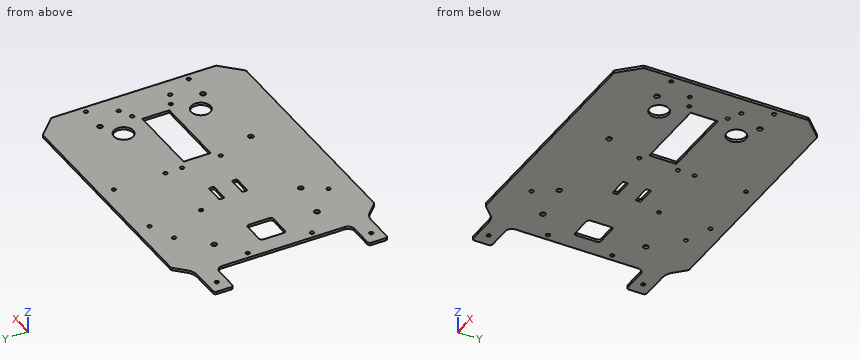
Autodesk Inventor part; units mm, degrees
ref_plane "РабПлоскость1" through (24.5, 0, 0) normal (0, 1, 0) x (1, 0, 0)
ref_plane "YZ Plane" through (0, 0, 0) normal (1, 0, 0) x (0, 1, 0)
ref_plane "XZ Plane" through (0, 0, 0) normal (0, 1, 0) x (-1, 0, 0)
sketch "Эскиз1" plane through (0, 0, 0) normal (0, 0, 1) x (1, 0, 0)
  line L0 (105, -79) -> (-105, -79)
  line L1 (-105, -79) -> (-105, 79)
  line L2 (-105, 79) -> (105, 79)
  line L3 (105, 79) -> (105, -79)
  line L4 (105, -79) -> (-105, 79) construction
  line L5 (-105, -79) -> (105, 79) construction
  point P0 (0, 0)
  dimension "d0" = 210
  dimension "d1" = 158
extrude "Выдавливание1" add sketch "Эскиз1" along normal blind 2
chamfer "Фаска1" distance 15 angle 45 4 edges at (105, -79, 1) (-105, -79, 1) (-105, 79, 1) (105, 79, 1)
fillet "Сопряжение1" radius 2 8 edges at (90, 79, 1) (105, 64, 1) (105, -64, 1) (90, -79, 1) (-90, -79, 1) (-105, -64, 1) (-90, 79, 1) (-105, 64, 1)
sketch "Эскиз2" plane through (0, 0, 2) normal (0, 0, 1) x (1, 0, 0)
  line L0 (-100, 40) -> (100, 40) construction
  line L1 (100, 40) -> (100, -40) construction
  line L2 (100, -40) -> (-100, -40) construction
  line L3 (-100, -40) -> (-100, 40) construction
  line L4 (-100, 40) -> (100, -40) construction
  line L5 (100, 40) -> (-100, -40) construction
  circle A0 centre (100, -40) radius 1.5
  circle A1 centre (100, 40) radius 1.5
  point P0 (0, 0)
  dimension "d8" = 200
  dimension "d9" = 80
  dimension "d10" = 3
  dimension "d13" = 3
extrude "фонарь" cut sketch "Эскиз2" against normal blind 2
sketch "Эскиз3" plane through (0, 0, 2) normal (0, 0, 1) x (1, 0, 0)
  line L0 (-90, 20) -> (90, 20) construction
  line L1 (90, 20) -> (90, -20) construction
  line L2 (90, -20) -> (-90, -20) construction
  line L3 (-90, -20) -> (-90, 20) construction
  line L4 (-90, 20) -> (90, -20) construction
  line L5 (90, 20) -> (-90, -20) construction
  circle A0 centre (90, -20) radius 1.5
  circle A1 centre (90, 20) radius 1.5
  point P0 (0, 0)
  dimension "d16" = 180
  dimension "d17" = 40
  dimension "d18" = 3
  dimension "d19" = 3
extrude "камера" cut sketch "Эскиз3" against normal blind 2
sketch "Эскиз4" plane through (0, 0, 2) normal (0, 0, 1) x (1, 0, 0)
  line L0 (-80, 40) -> (80, 40) construction
  line L1 (80, 40) -> (80, -40) construction
  line L2 (80, -40) -> (-80, -40) construction
  line L3 (-80, -40) -> (-80, 40) construction
  line L4 (-80, 40) -> (80, -40) construction
  line L5 (80, 40) -> (-80, -40) construction
  circle A0 centre (80, -40) radius 2
  circle A1 centre (-80, -40) radius 2
  circle A2 centre (-80, 40) radius 2
  circle A3 centre (80, 40) radius 2
  point P0 (0, 0)
  dimension "d22" = 160
  dimension "d23" = 80
  dimension "d24" = 4
  dimension "d25" = 4
  dimension "d26" = 4
  dimension "d27" = 4
extrude "крепление" cut sketch "Эскиз4" against normal blind 2
sketch "Эскиз6" plane through (0, 0, 2) normal (0, 0, 1) x (1, 0, 0)
  line L0 (-40, 68) -> (10, 68) construction
  line L1 (10, 68) -> (10, 28) construction
  line L2 (10, 28) -> (-40, 28) construction
  line L3 (-40, 28) -> (-40, 68) construction
  line L4 (-40, 68) -> (10, 28) construction
  line L5 (10, 68) -> (-40, 28) construction
  line L6 (-105, 63.1716) -> (-105, -63.1716) construction
  circle A0 centre (-80, 40) radius 2 construction
  circle A1 centre (10, 28) radius 1.5
  circle A2 centre (-40, 28) radius 1.5
  circle A3 centre (-40, 68) radius 1.5
  circle A4 centre (10, 68) radius 1.5
  point P0 (0, 0)
  point P1 (-15, 48)
  dimension "d46" = 50
  dimension "d47" = 40
  dimension "d48" = 65
  dimension "d49" = 30
  dimension "d50" = 3
  dimension "d51" = 3
  dimension "d52" = 3
  dimension "d53" = 3
extrude "Bullet" cut sketch "Эскиз6" against normal blind 10
sketch "Эскиз7" plane through (0, 0, 0) normal (0, 0, -1) x (-1, 0, 0)
  line L0 (105, -63.1716) -> (105, 63.1716) construction
  circle A0 centre (-20, -44) radius 2
  circle A1 centre (50, -44) radius 2
  line L1 (-89.1716, -79) -> (89.1716, -79)
  circle A2 centre (80, -40) radius 2
  point P0 (0, 0)
  dimension "d58" = 4
  dimension "d59" = 4
  dimension "d153" = 35
  dimension "d154" = 35
  dimension "d155" = 55
  dimension "d156" = 70
extrude "АКБ" cut sketch "Эскиз7" against normal blind 10 contours A0 | A1
sketch "Эскиз8" plane through (0, 0, 0) normal (0, 0, -1) x (-1, 0, 0)
  line L0 (-100, -25) -> (100, -25) construction
  line L1 (100, -25) -> (100, 25) construction
  line L2 (100, 25) -> (-100, 25) construction
  line L3 (-100, 25) -> (-100, -25) construction
  line L4 (-100, -25) -> (100, 25) construction
  line L5 (100, -25) -> (-100, 25) construction
  circle A0 centre (100, 25) radius 1.5
  circle A1 centre (100, -25) radius 1.5
  point P0 (0, 0)
  dimension "d65" = 200
  dimension "d66" = 50
  dimension "d67" = 3
  dimension "d68" = 3
extrude "Дисплей" cut sketch "Эскиз8" against normal blind 10
sketch "Эскиз9" plane through (0, 0, 0) normal (0, 0, -1) x (-1, 0, 0)
  line L0 (-24.5, -10.5) -> (-65.5, 10.5) construction
  line L1 (-65.5, -10.5) -> (-24.5, 10.5) construction
  line L2 (-10, -15) -> (-80, -15) construction
  line L3 (-80, -15) -> (-80, 15) construction
  line L4 (-80, 15) -> (-10, 15) construction
  line L5 (-10, 15) -> (-10, -15) construction
  line L6 (-10, -15) -> (-80, 15) construction
  line L7 (-80, -15) -> (-10, 15) construction
  circle A0 centre (-80, 40) radius 2 construction
  circle A1 centre (-80, 15) radius 1.5
  circle A2 centre (-80, -15) radius 1.5
  circle A3 centre (-10, -15) radius 1.5
  circle A4 centre (-10, 15) radius 1.5
  line L8 (-74, 10.5) -> (-16, 10.5)
  line L9 (-16, 10.5) -> (-16, -10.5)
  line L10 (-16, -10.5) -> (-74, -10.5)
  line L11 (-74, -10.5) -> (-74, 10.5)
  line L12 (-74, 10.5) -> (-16, -10.5) construction
  line L13 (-16, 10.5) -> (-74, -10.5) construction
  point P0 (0, 0)
  point P1 (-45, 0)
  point P2 (-45, 0)
  dimension "d71" = 41
  dimension "d72" = 21
  dimension "d73" = 70
  dimension "d74" = 30
  dimension "d75" = 0
  dimension "d76" = 3
  dimension "d77" = 3
  dimension "d78" = 3
  dimension "d79" = 3
  dimension "d82" = 41
  dimension "d157" = 58
  dimension "d158" = 21
extrude "Серво" cut sketch "Эскиз9" against normal blind 10
sketch "Эскиз10" plane through (0, 0, 0) normal (0, 0, -1) x (-1, 0, 0)
  line L0 (91, -10) -> (71, -10)
  line L1 (71, -10) -> (71, 10)
  line L2 (71, 10) -> (91, 10)
  line L3 (91, 10) -> (91, -10)
  line L4 (91, -10) -> (71, 10) construction
  line L5 (71, -10) -> (91, 10) construction
  line L6 (105, -63.1716) -> (105, 63.1716)
  point P0 (0, 0)
  point P1 (81, 0)
  point P2 (81, 0)
  dimension "d88" = 20
  dimension "d89" = 20
  dimension "d90" = 14
extrude "Для кабелей" cut sketch "Эскиз10" against normal blind 10
fillet "Сопряжение3" radius 2 4 edges at (-71, 10, 1) (-71, -10, 1) (-91, -10, 1) (-91, 10, 1)
sketch "Эскиз11" plane through (0, 0, 0) normal (0, 0, -1) x (-1, 0, 0)
  line L0 (70, -60) -> (120, -60) construction
  circle A0 centre (120, -60) radius 1.5
  line L1 (105, -63.1716) -> (105, 63.1716)
  circle A1 centre (80, -40) radius 2
  line L2 (130, -67.5) -> (60, -67.5)
  line L3 (60, -67.5) -> (60, -52.5)
  line L4 (60, -52.5) -> (130, -52.5)
  line L5 (130, -52.5) -> (130, -67.5)
  line L6 (130, -67.5) -> (60, -52.5) construction
  line L7 (60, -67.5) -> (130, -52.5) construction
  circle A2 centre (60, -60) radius 1.5
  point P0 (0, 0)
  point P1 (95, -60)
  dimension "d94" = 50
  dimension "d96" = 3
  dimension "d98" = 20
  dimension "d99" = 70
  dimension "d100" = 15
  dimension "d126" = 3
  dimension "d127" = 60
  dimension "d128" = 25
extrude "Выдавливание10" add sketch "Эскиз11" against normal blind 2 contours L2 L3 A2 L4 L5 | L3 A2 picked at (60.1113, -59.5125)
extrude "Выдавливание11" cut sketch "Эскиз11" against normal blind 2 contours A2 L3 | L3 A2
fillet "Сопряжение4" radius 2 2 edges at (-130, -52.5, 1) (-130, -67.5, 1)
fillet "Сопряжение5" radius 12 1 edges at (-101.5, -67.5, 1)
fillet "Сопряжение6" radius 5 1 edges at (-105, -52.5, 1)
ref_plane "РабПлоскость1" through (24.5, 0, 0) normal (0, 1, 0) x (1, 0, 0)
mirror "Зеркальное отражение1" about plane through (24.5, 0, 0) normal (0, 1, 0) of "Выдавливание10"
mirror "Зеркальное отражение2" about plane through (24.5, 0, 0) normal (0, 1, 0) of "Выдавливание11"
mirror "Зеркальное отражение3" about plane through (24.5, 0, 0) normal (0, 1, 0) of "Сопряжение4", "Сопряжение5", "Сопряжение6"
sketch "Эскиз13" plane through (0, 0, 0) normal (0, 0, -1) x (-1, 0, 0)
  line L0 (20, 11) -> (35, 11)
  line L1 (35, 11) -> (35, 7)
  line L2 (35, 7) -> (20, 7)
  line L3 (20, 7) -> (20, 11)
  line L4 (20, -7) -> (35, -7)
  line L5 (35, -7) -> (35, -11)
  line L6 (35, -11) -> (20, -11)
  line L7 (20, -11) -> (20, -7)
  line L8 (105, -47.5) -> (105, 47.5)
  point P0 (0, 0)
  point P1 (105, -63.1716)
  point P2 (105, 63.1716)
  dimension "d108" = 15
  dimension "d109" = 4
  dimension "d110" = 15
  dimension "d111" = 4
  dimension "d112" = 7
  dimension "d113" = 7
  dimension "d114" = 70
extrude "Выдавливание12" cut sketch "Эскиз13" against normal blind 2
fillet "Сопряжение7" radius 1 8 edges at (-20, -7, 1) (-20, 11, 1) (-35, -11, 1) (-35, 7, 1) (-20, -11, 1) (-20, 7, 1) (-35, 11, 1) (-35, -7, 1)
sketch "Эскиз14" plane through (0, 0, 0) normal (0, 0, -1) x (-1, 0, 0)
  circle A0 centre (-65, -30) radius 7.5
  circle A1 centre (-65, 30) radius 7.5
  circle A2 centre (-80, 15) radius 1.5
  circle A3 centre (-80, -15) radius 1.5
  point P0 (0, 0)
  dimension "d118" = 15
  dimension "d119" = 15
  dimension "d120" = 15
  dimension "d121" = 15
  dimension "d122" = 15
  dimension "d123" = 15
extrude "Выдавливание13" cut sketch "Эскиз14" against normal blind 2 contours A0 | A1
sketch "Эскиз15" plane through (0, 0, 2) normal (0, 0, 1) x (1, 0, 0)
  line L0 (100, -15) -> (30, -15) construction
  line L1 (30, -15) -> (30, 15) construction
  line L2 (30, 15) -> (100, 15) construction
  line L3 (100, 15) -> (100, -15) construction
  line L4 (100, -15) -> (30, 15) construction
  line L5 (30, -15) -> (100, 15) construction
  line L6 (105, -63.1716) -> (105, 63.1716) construction
  circle A0 centre (100, 15) radius 1.5
  circle A1 centre (30, 15) radius 1.5
  circle A2 centre (30, -15) radius 1.5
  circle A3 centre (100, -15) radius 1.5
  line L7 (85.5, -10.5) -> (44.5, -10.5)
  line L8 (44.5, -10.5) -> (44.5, 10.5)
  line L9 (44.5, 10.5) -> (85.5, 10.5)
  line L10 (85.5, -10.5) -> (44.5, 10.5) construction
  line L11 (44.5, -10.5) -> (85.5, 10.5) construction
  line L12 (90.5, -3.5) -> (85.5, -3.5)
  line L13 (85.5, 3.5) -> (90.5, 3.5)
  line L14 (90.5, 3.5) -> (90.5, -3.5)
  line L15 (90.5, -3.5) -> (80.5, 3.5) construction
  line L16 (80.5, -3.5) -> (90.5, 3.5) construction
  line L17 (85.5, 10.5) -> (85.5, 3.5)
  line L18 (85.5, -3.5) -> (85.5, -10.5)
  point P0 (0, 0)
  point P1 (65, 0)
  point P2 (65, 0)
  point P3 (85.5, 0)
  point P4 (65, 0)
  point P5 (85.5, 0)
  point P6 (85.5, 0)
  dimension "d129" = 70
  dimension "d130" = 30
  dimension "d131" = 5
  dimension "d132" = 3
  dimension "d133" = 3
  dimension "d134" = 3
  dimension "d135" = 3
  dimension "d136" = 41
  dimension "d137" = 21
  dimension "d138" = 10
  dimension "d139" = 7
  dimension "d141" = 7
  dimension "d142" = 7
  dimension "d143" = 41
  dimension "d144" = 7
sketch "Эскиз16" plane through (0, 0, 2) normal (0, 0, 1) x (1, 0, 0)
  circle A0 centre (100, 15) radius 1.5
  circle A1 centre (80, 15) radius 1.5
  line L0 (100, 16.5) -> (80, 16.5)
  line L1 (80, 16.5) -> (80, 13.5)
  line L2 (80, 13.5) -> (100, 13.5)
  line L3 (100, 13.5) -> (100, 16.5)
  circle A2 centre (100, -15) radius 1.5
  circle A3 centre (80, -15) radius 1.5
  line L4 (100, -13.5) -> (80, -13.5)
  line L5 (80, -13.5) -> (80, -16.5)
  line L6 (80, -16.5) -> (100, -16.5)
  line L7 (100, -16.5) -> (100, -13.5)
  circle A4 centre (30, -15) radius 1.5
  circle A5 centre (10, -15) radius 1.5
  line L8 (30, -13.5) -> (10, -13.5)
  line L9 (10, -13.5) -> (10, -16.5)
  line L10 (10, -16.5) -> (30, -16.5)
  line L11 (30, -16.5) -> (30, -13.5)
  circle A6 centre (30, 15) radius 1.5
  circle A7 centre (10, 15) radius 1.5
  line L12 (30, 16.5) -> (10, 16.5)
  line L13 (10, 16.5) -> (10, 13.5)
  line L14 (10, 13.5) -> (30, 13.5)
  line L15 (30, 13.5) -> (30, 16.5)
  point P0 (0, 0)
equation "\"d119\" = d118"
equation "\"d120\" = d121"
equation "\"d123\" = d122"
properties part number "baseUp"
The model under review builds one solid part; all positions refer to its coordinate system, in mm. Round coordinates to 2 decimals unless told otherwise and drop trailing zeros. Order: outer loops, then holes, each group sorted by start corner. A loop starts at its lowest first (then second) coordinate and runs counter-clockwise, first axis right, second up. Notation, with made-up numbers: (24.25, 33) -> (32.25, 33) arc R25 cw to (32.25, 61) -> close; hole circle Ø3 at (-19, 38.5). An arc over 180 degrees is marked (long way). Use CSV: the item, a comma, the result in double quotes. Start each with the question number.
(1) Insertion check: pin 1 (24 mm diameter, centred on x = 65, y = -30, fed in from -Z); pin 2 (1 mm diameter, centred on x = -112, z = 0.5, fed in from +Y); pin 3 (0.6 mm diameter, centred on y = -9.5, z = 0.5, fed in from -X). Each pin has a flat end and moves straight along its axis. Give the tip position at first contact, or say it passes through.
(2) Consider section B-B on y = 34. Write out the cut boundary in (x, z), and give its area (3 significant figures).
(3) Wall thickness on probe 1 along Y at (x, z) = (80, 0.85); probe 2 along Y at (x, z) = (-80, 1.5); probe 3 along Y at (x, z) = (-40, 0.4): over which ranges is each line inside the solid? List them lowest first. Write a range as from..to.
(4) Consider section C-C on z = 1.25. State how many separate pieces and enclosed holes the cut face has, and give its area (3 significant figures).
(5) Consider section A-A on x = 27. Write out the cut boundary in (y, z), and give its area (3 significant figures).
Responses:
1,pin 1,"z = 0"
1,pin 2,"y = 67.5"
1,pin 3,"x = -105"
2,outline,"(-105, 0) -> (58.66, 0) -> (58.66, 2) -> (-105, 2) -> close; (71.34, 0) -> (105, 0) -> (105, 2) -> (71.34, 2) -> close"
2,area,"395 mm²"
3,probe 1,"-79..-42, -38..-16.5, -13.5..13.5, 16.5..38, 42..79"
3,probe 2,"-79..-42, -38..-10, 10..38, 42..79"
3,probe 3,"-79..26.5, 29.5..66.5, 69.5..79"
4,separate pieces,"1"
4,enclosed holes,"30"
4,area,"31,200 mm²"
5,outline,"(-79, 0) -> (-10.5, 0) -> (-10.5, 2) -> (-79, 2) -> close; (10.5, 0) -> (79, 0) -> (79, 2) -> (10.5, 2) -> close"
5,area,"274 mm²"
